Input: dimensioned drawing with shaded views. Units: mm. Origin: part minimum x, y, z. A direction names the side the tool comes from. Coordinates: 2 decimals unless noted, no trailing zeros. Order: outer loops, then holes, each group sorted by start corner. A loop starts at its lowest first (then second) coordinate and runs counter-clockwise, first axis right, second up.
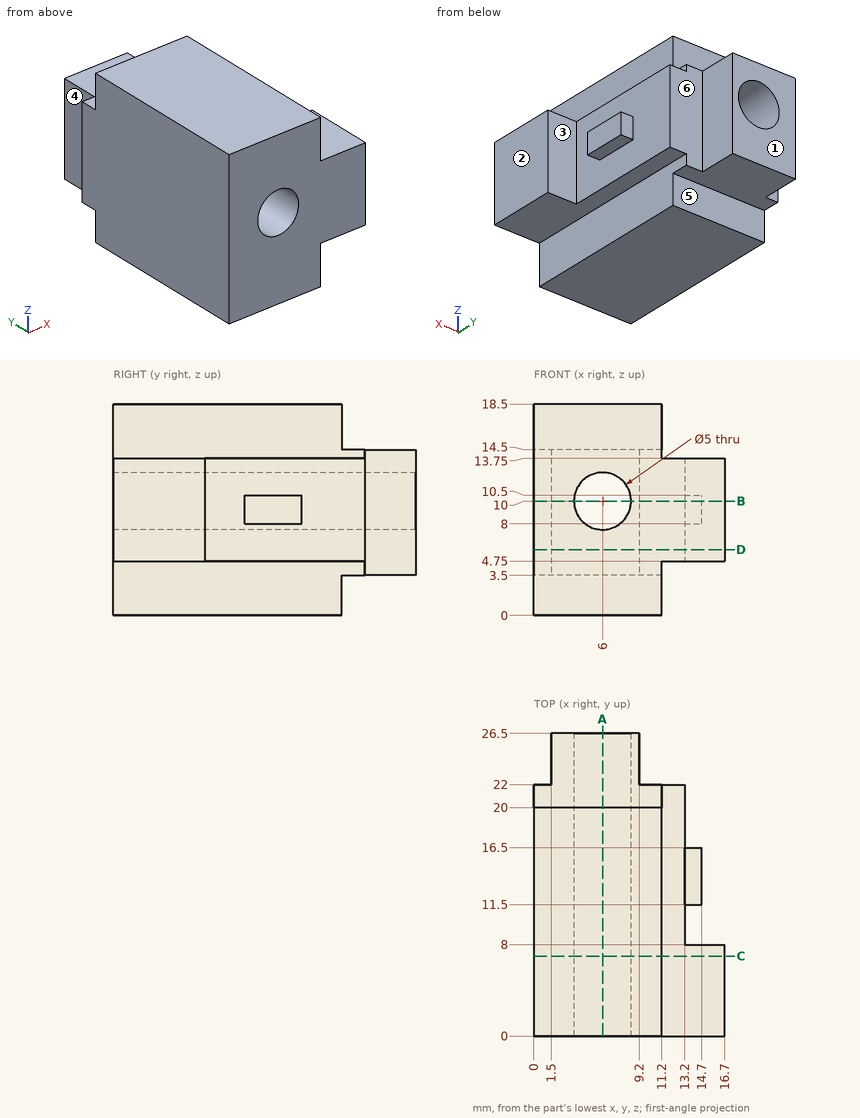
1. Section query A-A on x = 6. Return loops of the section in (y, z).
Findings:
outline: (0, 0) - (20, 0) - (20, 3.5) - (26.5, 3.5) - (26.5, 7.5) - (0, 7.5) - close; (0, 12.5) - (26.5, 12.5) - (26.5, 14.5) - (20, 14.5) - (20, 18.5) - (0, 18.5) - close
2. Pin query (flat end, axial travel): P1, Ø2, axis at x = 3.5, y = 24.5, coming from the -Z side; P2, Ø0.8, axis at x = 14, y = 15, coming from the +Z side; P3, Ø4.5, axis at y = 14, z = 7.5, coming from the +X side. Return the tip coordinate at first contact, or that it passes through.
Findings:
P1: stops at z = 3.5
P2: stops at z = 10.5
P3: stops at x = 14.7
3. Access query for the marked faces 4, 5 and 6. Directions: +Z, -Z, +X, -X, +Y, -Y. A direction counts if a zero-diameter tool reaches every point of the face in a straight line with its end or side. Return the directions, or none.
Findings:
face 4: +Z, -Z, -X, +Y
face 5: -Z, +X, -X, +Y
face 6: +Z, -Z, +X, +Y
4. Section query B-B on z = 10. Return loops of the section in (x, y), plus the area to 3 significant figures.
Findings:
outline: (0, 0) - (3.5, 0) - (3.5, 26.5) - (1.5, 26.5) - (1.5, 22) - (0, 22) - close; (8.5, 0) - (16.7, 0) - (16.7, 8) - (13.2, 8) - (13.2, 11.5) - (14.7, 11.5) - (14.7, 16.5) - (13.2, 16.5) - (13.2, 22) - (9.2, 22) - (9.2, 26.5) - (8.5, 26.5) - close
area: 228 mm2
5. Section query D-D on z = 5.75. Return loops of the section in (x, y), plus the area to 3 significant figures.
Findings:
outline: (0, 0) - (16.7, 0) - (16.7, 8) - (13.2, 8) - (13.2, 22) - (9.2, 22) - (9.2, 26.5) - (1.5, 26.5) - (1.5, 22) - (0, 22) - close
area: 353 mm2
6. Ray query, line 1 (Z direction, x = 4, y = 20.75); line 2 (Y direction, x = 15, z = 5.25); line 3 (X direction, y = 1.25, z = 14.75). Return the intervals inside material, ascending.
Findings:
line 1: z = 3.5 to 8.5, 11.5 to 14.5
line 2: y = 0 to 8
line 3: x = 0 to 11.2
7. Section query C-C on y = 7. Return loops of the section in (x, z).
Findings:
outline: (0, 0) - (11.2, 0) - (11.2, 4.75) - (16.7, 4.75) - (16.7, 13.75) - (11.2, 13.75) - (11.2, 18.5) - (0, 18.5) - close; hole circle Ø5 at (6, 10)
8. Draft query along Y for the marked faces 1, 2 and 3. Return one class per face: released by +Y, released by -Y, zero draft, split by the parting line, or undercut.
Findings:
face 1: released by +Y
face 2: zero draft
face 3: undercut
